from build123d import *

# Parameters (mm, degrees)
F0_R      = 17
F1_DEPTH  = 3
F3_R      = 2.99999
F5_R      = 12.4526743877
F6_DEPTH  = 0.5588
F7_R      = 5
F8_DEPTH  = 1.143
F10_R     = 2.25
F11_DEPTH = 25.4
F13_DEPTH = 0.1
F14_R     = 1.5
F15_DEPTH = 1


# Not quite as in the source:
# - a fillet or chamfer is up to 0.001 mm smaller than in the source, because OpenCascade refuses the exact size


with BuildPart() as f1:
    # F0 (on Front) → F1 (new body)
    with BuildSketch(Plane.XZ):
        Circle(F0_R)
    extrude(amount=F1_DEPTH)

    # F3 (radius 3 in the source; OpenCascade refuses exactly that, so slightly less here)
    f3_edges = [f1.edges().sort_by_distance(p)[0] for p in [
        (-17, -3, 0),
    ]]
    fillet(f3_edges, radius=F3_R)

    # F5 (on face) → F6 (cut)
    with BuildSketch(Plane.XZ.offset(3)):
        Circle(F5_R)
    extrude(amount=-F6_DEPTH, mode=Mode.SUBTRACT)

    # F7 (on face) → F8 (join)
    with BuildSketch(Plane.XZ.offset(3)):
        Circle(F7_R)
    extrude(amount=-F8_DEPTH)

    # F10 (on face) → F11 (cut)
    with BuildSketch(Plane.XZ.offset(3)):
        with BuildLine():
            ThreePointArc((8.6139610307, -6.3639610307), (7.2249987535, -4.2852320825), (4.772970773, -4.772970773))
            ThreePointArc((4.772970773, -4.772970773), (5.5029233079, -8.4426899788), (8.6139610307, -6.3639610307))
        make_face()
        with BuildLine():
            ThreePointArc((2.25, -9), (1.5909902577, -7.4090097423), (0, -6.75))
            ThreePointArc((0, -6.75), (-1.5909902577, -10.5909902577), (2.25, -9))
        make_face()
        with BuildLine():
            ThreePointArc((-4.1139610307, -6.3639610307), (-4.2852320825, -5.5029233079), (-4.772970773, -4.772970773))
            ThreePointArc((-4.772970773, -4.772970773), (-8.4426899788, -7.2249987535), (-4.1139610307, -6.3639610307))
        make_face()
        with BuildLine():
            ThreePointArc((10.9506839843, 0), (9, 1.9506839843), (7.0493160157, 0))
            ThreePointArc((7.0493160157, 0), (9, -1.9506839843), (10.9506839843, 0))
        make_face()
        with Locations((-9, 0)):
            Circle(F10_R)
        with BuildLine():
            ThreePointArc((-4.1139610307, 6.3639610307), (-8.4426899788, 7.2249987535), (-4.772970773, 4.772970773))
            ThreePointArc((-4.772970773, 4.772970773), (-4.2852320825, 5.5029233079), (-4.1139610307, 6.3639610307))
        make_face()
        with BuildLine():
            ThreePointArc((2.25, 9), (-1.5909902577, 10.5909902577), (0, 6.75))
            ThreePointArc((0, 6.75), (1.5909902577, 7.4090097423), (2.25, 9))
        make_face()
        with BuildLine():
            ThreePointArc((8.6139610307, 6.3639610307), (5.5029233079, 8.4426899788), (4.772970773, 4.772970773))
            ThreePointArc((4.772970773, 4.772970773), (7.2249987535, 4.2852320825), (8.6139610307, 6.3639610307))
        make_face()
    extrude(amount=-F11_DEPTH, mode=Mode.SUBTRACT)

    # F12 (on face) → F13 (join)
    with BuildSketch(Plane.XZ.offset(3)):
        with BuildLine():
            Line((-2.1213203436, 2.1213203436), (-1.767766953, 1.767766953))
            ThreePointArc((-1.767766953, 1.767766953), (-1.6593805773, 1.9299786274), (-1.6213203436, 2.1213203436))
            ThreePointArc((-1.6213203436, 2.1213203436), (-1.9299786274, 2.5832601098), (-2.4748737342, 2.4748737342))
            Line((-2.4748737342, 2.4748737342), (-2.1213203436, 2.1213203436))
        make_face()
        with BuildLine():
            ThreePointArc((-2.4748737342, 2.4748737342), (-2.4748737342, 1.767766953), (-1.767766953, 1.767766953))
            Line((-1.767766953, 1.767766953), (-2.1213203436, 2.1213203436))
            Line((-2.1213203436, 2.1213203436), (-2.4748737342, 2.4748737342))
        make_face()
        with BuildLine():
            Line((0, 3), (0, 3.5))
            ThreePointArc((0, 3.5), (-0.5, 3), (0, 2.5))
            Line((0, 2.5), (0, 3))
        make_face()
        with BuildLine():
            ThreePointArc((0.5, 3), (0.3535533906, 3.3535533906), (0, 3.5))
            Line((0, 3.5), (0, 3))
            Line((0, 3), (0, 2.5))
            ThreePointArc((0, 2.5), (0.3535533906, 2.6464466094), (0.5, 3))
        make_face()
        with BuildLine():
            ThreePointArc((2.6213203436, -2.1213203436), (2.3126620597, -1.6593805773), (1.767766953, -1.767766953))
            Line((1.767766953, -1.767766953), (2.1213203436, -2.1213203436))
            Line((2.1213203436, -2.1213203436), (2.4748737342, -2.4748737342))
            ThreePointArc((2.4748737342, -2.4748737342), (2.5832601098, -2.3126620597), (2.6213203436, -2.1213203436))
        make_face()
        with BuildLine():
            Line((2.1213203436, -2.1213203436), (1.767766953, -1.767766953))
            ThreePointArc((1.767766953, -1.767766953), (1.767766953, -2.4748737342), (2.4748737342, -2.4748737342))
            Line((2.4748737342, -2.4748737342), (2.1213203436, -2.1213203436))
        make_face()
        with BuildLine():
            ThreePointArc((-3.5, 0), (-3, -0.5), (-2.5, 0))
            Line((-2.5, 0), (-3, 0))
            Line((-3, 0), (-3.5, 0))
        make_face()
        with BuildLine():
            Line((-3, 0), (-2.5, 0))
            ThreePointArc((-2.5, 0), (-3, 0.5), (-3.5, 0))
            Line((-3.5, 0), (-3, 0))
        make_face()
        with BuildLine():
            Line((-2.1213203436, -2.1213203436), (-1.767766953, -1.767766953))
            ThreePointArc((-1.767766953, -1.767766953), (-2.4748737342, -1.767766953), (-2.4748737342, -2.4748737342))
            Line((-2.4748737342, -2.4748737342), (-2.1213203436, -2.1213203436))
        make_face()
        with BuildLine():
            ThreePointArc((-1.6213203436, -2.1213203436), (-1.6593805773, -1.9299786274), (-1.767766953, -1.767766953))
            Line((-1.767766953, -1.767766953), (-2.1213203436, -2.1213203436))
            Line((-2.1213203436, -2.1213203436), (-2.4748737342, -2.4748737342))
            ThreePointArc((-2.4748737342, -2.4748737342), (-1.9299786274, -2.5832601098), (-1.6213203436, -2.1213203436))
        make_face()
        with BuildLine():
            ThreePointArc((0.5, -3), (0.3535533906, -2.6464466094), (0, -2.5))
            Line((0, -2.5), (0, -3))
            Line((0, -3), (0, -3.5))
            ThreePointArc((0, -3.5), (0.3535533906, -3.3535533906), (0.5, -3))
        make_face()
        with BuildLine():
            Line((0, -3), (0, -2.5))
            ThreePointArc((0, -2.5), (-0.5, -3), (0, -3.5))
            Line((0, -3.5), (0, -3))
        make_face()
        with BuildLine():
            Line((3, 0), (2.5, 0))
            ThreePointArc((2.5, 0), (3, -0.5), (3.5, 0))
            Line((3.5, 0), (3, 0))
        make_face()
        with BuildLine():
            ThreePointArc((3.5, 0), (3, 0.5), (2.5, 0))
            Line((2.5, 0), (3, 0))
            Line((3, 0), (3.5, 0))
        make_face()
        with BuildLine():
            Line((2.1213203436, 2.1213203436), (1.767766953, 1.767766953))
            ThreePointArc((1.767766953, 1.767766953), (2.3126620597, 1.6593805773), (2.6213203436, 2.1213203436))
            ThreePointArc((2.6213203436, 2.1213203436), (2.5832601098, 2.3126620597), (2.4748737342, 2.4748737342))
            Line((2.4748737342, 2.4748737342), (2.1213203436, 2.1213203436))
        make_face()
        with BuildLine():
            ThreePointArc((2.4748737342, 2.4748737342), (1.767766953, 2.4748737342), (1.767766953, 1.767766953))
            Line((1.767766953, 1.767766953), (2.1213203436, 2.1213203436))
            Line((2.1213203436, 2.1213203436), (2.4748737342, 2.4748737342))
        make_face()
    extrude(amount=F13_DEPTH)

    # F14 (on face) → F15 (join)
    with BuildSketch(Plane.XZ.offset(3)):
        Circle(F14_R)
    extrude(amount=F15_DEPTH)


solid = f1.part
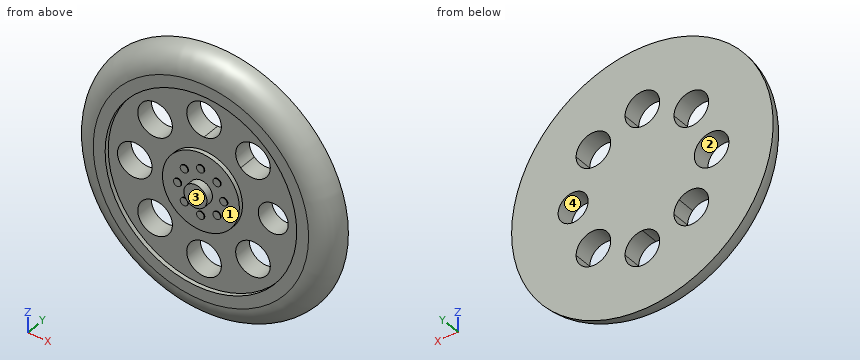
For this review, take the finished solid that the model builds, in its own axes (mm). Face numbers are marked on the shaded views. A direction names the side the tool comes from. Give positions to 0.01 mm unless a question says otherwise; leave off trailing zeros. Answer as a JSON object with one key per item and string values. Group by question number.
Q1. Mouldability with a two-part tool opening along Z and no side actions: class the marked faces 3 and 4 as +Z half, -Z half, draft (parallel to the pull), parting line (faces both ways), or undercut.
Q2. Add section A-A on y = -1.3. Give the number of separate pieces and of enclosed holes in the cut face, and give its area (3 significant figures).
Q3. Insertion check: P1, Ø0.8, axis at x = 2, z = 2, coming from the -Y side; P2, Ø8, axis at x = -7, z = -11, coming from the -Y side; P3, Ø5, axis at x = 0, z = 9, coming from the -Y side; P4, Ø4, axis at x = 6.36, z = -6.36, coming from the +Y side. Each pin has a flat end and moves straight along its axis. Give the tip position at first contact, or say it passes through.
Q4. Tool access review of the marked faces 1 and 2: name each direction out of +Z, -Z, +X, -X, +Y, -Y from which nothing blocks a thin tool from reaching the whole face with its end or side.
Q5. For probe 1 along X at (y, z) = (-0.65, 7); probe 2 along X at (y, z) = (-2, 7.5); probe 3 along Z at (x, y) = (6.5, -0.35), list the stretches that pass through material, from the lowest coordinate up. Write a range as [from, to].
Checked values:
{
 "1": {"face 3": "draft", "face 4": "undercut"},
 "2": {"separate pieces": "1", "enclosed holes": "8", "area": "753 mm²"},
 "3": {"P1": "y = -3.1", "P2": "y = -3", "P3": "y = -2.44", "P4": "through"},
 "4": {"face 1": "-Y", "face 2": "+Y, -Y"},
 "5": {"probe 1": "[-15.41, -8.52], [-4.21, -1.03], [1.03, 4.21], [8.52, 15.41]", "probe 2": "[-14.4, -8.31], [-4.42, -1.68], [1.68, 4.42], [8.31, 14.4]", "probe 3": "[-15.69, -8.61], [-4.12, 4.12], [8.61, 15.69]"}
}
